```python
from build123d import *

# Parameters (mm, degrees)
MODEL_R             = 5
BOSS_EXTRUDE1_DEPTH = 500


with BuildPart() as part:
    # Model → Boss-Extrude1 (new body)
    with BuildSketch(Plane.XY):
        with BuildLine():
            Line((7.8, 0), (7.8, -4.021825407))
            ThreePointArc((7.8, -4.021825407), (8.10448187, -5.552559136), (8.971572875, -6.850252532))
            Line((8.971572875, -6.850252532), (13.121320343, -11))
            Line((13.121320343, -11), (15.8, -11))
            ThreePointArc((15.8, -11), (16.224264069, -10.824264069), (16.4, -10.4))
            Line((16.4, -10.4), (16.4, -6.8))
            ThreePointArc((16.4, -6.8), (16.575735931, -6.375735931), (17, -6.2))
            Line((17, -6.2), (18.4, -6.2))
            ThreePointArc((18.4, -6.2), (18.824264069, -6.375735931), (19, -6.8))
            Line((19, -6.8), (19, -7.2))
            Line((19, -7.2), (19.4, -7.2))
            ThreePointArc((19.4, -7.2), (19.824264068, -7.375735931), (20, -7.8))
            Line((20, -7.8), (20, -17))
            ThreePointArc((20, -17), (19.121320343, -19.121320343), (17, -20))
            Line((17, -20), (7.8, -20))
            ThreePointArc((7.8, -20), (7.375735931, -19.824264069), (7.2, -19.4))
            ThreePointArc((7.2, -19.4), (7.082842712, -19.117157287), (6.8, -19))
            ThreePointArc((6.8, -19), (6.375735931, -18.824264069), (6.2, -18.4))
            Line((6.2, -18.4), (6.2, -16.999999999))
            ThreePointArc((6.2, -16.999999999), (6.375735931, -16.575735931), (6.8, -16.4))
            Line((6.8, -16.4), (10.4, -16.4))
            ThreePointArc((10.4, -16.4), (10.824264069, -16.224264069), (11, -15.8))
            Line((11, -15.8), (11, -13.369848481))
            ThreePointArc((11, -13.369848481), (10.954327719, -13.140238421), (10.824264069, -12.945584412))
            Line((10.824264069, -12.945584412), (6.850252532, -8.971572875))
            ThreePointArc((6.850252532, -8.971572875), (5.552559136, -8.10448187), (4.021825407, -7.8))
            Line((4.021825407, -7.8), (0, -7.8))
            Line((0, -7.8), (-4.021825407, -7.8))
            ThreePointArc((-4.021825407, -7.8), (-5.552559136, -8.10448187), (-6.850252532, -8.971572875))
            Line((-6.850252532, -8.971572875), (-10.824264069, -12.945584412))
            ThreePointArc((-10.824264069, -12.945584412), (-10.954327719, -13.140238421), (-11, -13.369848481))
            Line((-11, -13.369848481), (-11, -15.8))
            ThreePointArc((-11, -15.8), (-10.824264069, -16.224264069), (-10.4, -16.4))
            Line((-10.4, -16.4), (-6.8, -16.4))
            ThreePointArc((-6.8, -16.4), (-6.375735931, -16.575735931), (-6.2, -16.999999999))
            Line((-6.2, -16.999999999), (-6.2, -18.4))
            ThreePointArc((-6.2, -18.4), (-6.375735931, -18.824264069), (-6.8, -19))
            ThreePointArc((-6.8, -19), (-7.082842712, -19.117157287), (-7.2, -19.4))
            ThreePointArc((-7.2, -19.4), (-7.375735931, -19.824264069), (-7.8, -20))
            Line((-7.8, -20), (-17, -20))
            ThreePointArc((-17, -20), (-19.121320343, -19.121320343), (-20, -17))
            Line((-20, -17), (-20, -7.8))
            ThreePointArc((-20, -7.8), (-19.824264069, -7.375735931), (-19.4, -7.2))
            Line((-19.4, -7.2), (-19, -7.2))
            Line((-19, -7.2), (-19, -6.8))
            ThreePointArc((-19, -6.8), (-18.824264069, -6.375735931), (-18.4, -6.2))
            Line((-18.4, -6.2), (-17, -6.2))
            ThreePointArc((-17, -6.2), (-16.575735931, -6.375735931), (-16.4, -6.8))
            Line((-16.4, -6.8), (-16.4, -10.4))
            ThreePointArc((-16.4, -10.4), (-16.224264069, -10.824264069), (-15.8, -11))
            Line((-15.8, -11), (-13.369848481, -11))
            ThreePointArc((-13.369848481, -11), (-13.140238421, -10.954327719), (-12.945584412, -10.824264069))
            Line((-12.945584412, -10.824264069), (-8.971572875, -6.850252532))
            ThreePointArc((-8.971572875, -6.850252532), (-8.10448187, -5.552559136), (-7.8, -4.021825407))
            Line((-7.8, -4.021825407), (-7.8, 0))
            Line((-7.8, 0), (-7.8, 4.021825407))
            ThreePointArc((-7.8, 4.021825407), (-8.10448187, 5.552559136), (-8.971572875, 6.850252532))
            Line((-8.971572875, 6.850252532), (-12.945584412, 10.824264069))
            ThreePointArc((-12.945584412, 10.824264069), (-13.140238421, 10.954327719), (-13.369848481, 11))
            Line((-13.369848481, 11), (-15.8, 11))
            ThreePointArc((-15.8, 11), (-16.224264069, 10.824264069), (-16.4, 10.4))
            Line((-16.4, 10.4), (-16.4, 6.8))
            ThreePointArc((-16.4, 6.8), (-16.575735931, 6.375735931), (-17, 6.2))
            Line((-17, 6.2), (-18.4, 6.2))
            ThreePointArc((-18.4, 6.2), (-18.824264069, 6.375735931), (-19, 6.8))
            Line((-19, 6.8), (-19, 7.2))
            Line((-19, 7.2), (-19.4, 7.2))
            ThreePointArc((-19.4, 7.2), (-19.824264069, 7.375735931), (-20, 7.8))
            Line((-20, 7.8), (-20, 17))
            ThreePointArc((-20, 17), (-19.121320343, 19.121320343), (-17, 20))
            Line((-17, 20), (-7.8, 20))
            ThreePointArc((-7.8, 20), (-7.375735931, 19.824264068), (-7.2, 19.4))
            Line((-7.2, 19.4), (-7.2, 19))
            Line((-7.2, 19), (-6.8, 19))
            ThreePointArc((-6.8, 19), (-6.375735931, 18.824264069), (-6.2, 18.4))
            Line((-6.2, 18.4), (-6.2, 16.999999999))
            ThreePointArc((-6.2, 16.999999999), (-6.375735931, 16.575735931), (-6.8, 16.4))
            Line((-6.8, 16.4), (-10.4, 16.4))
            ThreePointArc((-10.4, 16.4), (-10.824264069, 16.224264069), (-11, 15.8))
            Line((-11, 15.8), (-11, 13.369848481))
            ThreePointArc((-11, 13.369848481), (-10.954327719, 13.140238421), (-10.824264069, 12.945584412))
            Line((-10.824264069, 12.945584412), (-6.850252532, 8.971572875))
            ThreePointArc((-6.850252532, 8.971572875), (-5.552559136, 8.10448187), (-4.021825407, 7.8))
            Line((-4.021825407, 7.8), (0, 7.8))
            Line((0, 7.8), (4.021825407, 7.8))
            ThreePointArc((4.021825407, 7.8), (5.552559136, 8.10448187), (6.850252532, 8.971572875))
            Line((6.850252532, 8.971572875), (10.824264069, 12.945584412))
            ThreePointArc((10.824264069, 12.945584412), (10.954327719, 13.140238421), (11, 13.369848481))
            Line((11, 13.369848481), (11, 15.8))
            ThreePointArc((11, 15.8), (10.824264069, 16.224264069), (10.4, 16.4))
            Line((10.4, 16.4), (6.8, 16.4))
            ThreePointArc((6.8, 16.4), (6.375735931, 16.575735931), (6.2, 16.999999999))
            Line((6.2, 16.999999999), (6.2, 18.4))
            ThreePointArc((6.2, 18.4), (6.375735931, 18.824264069), (6.8, 19))
            Line((6.8, 19), (7.2, 19))
            Line((7.2, 19), (7.2, 19.4))
            ThreePointArc((7.2, 19.4), (7.375735931, 19.824264068), (7.8, 20))
            Line((7.8, 20), (17, 20))
            ThreePointArc((17, 20), (19.121320343, 19.121320343), (20, 17))
            Line((20, 17), (20, 7.8))
            ThreePointArc((20, 7.8), (19.824264068, 7.375735931), (19.4, 7.2))
            Line((19.4, 7.2), (19, 7.2))
            Line((19, 7.2), (19, 6.8))
            ThreePointArc((19, 6.8), (18.824264069, 6.375735931), (18.4, 6.2))
            Line((18.4, 6.2), (17, 6.2))
            ThreePointArc((17, 6.2), (16.575735931, 6.375735931), (16.4, 6.8))
            Line((16.4, 6.8), (16.4, 10.4))
            ThreePointArc((16.4, 10.4), (16.224264069, 10.824264069), (15.8, 11))
            Line((15.8, 11), (13.369848481, 11))
            ThreePointArc((13.369848481, 11), (13.140238421, 10.954327719), (12.945584412, 10.824264069))
            Line((12.945584412, 10.824264069), (8.971572875, 6.850252532))
            ThreePointArc((8.971572875, 6.850252532), (8.10448187, 5.552559136), (7.8, 4.021825407))
            Line((7.8, 4.021825407), (7.8, 0))
        make_face()
        Circle(MODEL_R, mode=Mode.SUBTRACT)
    extrude(amount=BOSS_EXTRUDE1_DEPTH)


solid = part.part
```
Input: part model. Units: mm. Frame: model coordinates. A direction names the side the tool comes from. Round coordinates to 2 decimals unless told otherwise and drop trailing zeros. Write each question's results on one line, items separated by ' | '.
Q1. Pin query (flat end, axial travel): P1, Ø0.7, axis at y = 17.5, z = 296.5, coming from the +X side; P2, Ø1.5, axis at x = 2, y = 3.5, coming from the -Z side; P3, Ø1, axis at y = -3.5, z = 246, coming from the +X side. Return the tip coordinate at first contact, or that it passes through.
Results:
P1: stops at x = 20 | P2: passes through | P3: stops at x = 7.8
Q2. Line query: line 1 along X through (y, z) = (14.5, 415.5); line 2 along Y through (x, z) = (0, 236); line 3 along X through (y, z) = (-3, 308). Output: solid intervals per line, ascending.
Results:
line 1: x = -20 to -11, 11 to 20 | line 2: y = -7.8 to -5, 5 to 7.8 | line 3: x = -7.8 to -4, 4 to 7.8
Q3. Access query for faces 1 (the face through (-7.8, 0, 246)), 2 (the face through (-12, 20, 246)), 3 (the face through (0, -7.8, 246)). Directions: +Z, -Z, +X, -X, +Y, -Y. A direction counts if a zero-diameter tool reaches every point of the face in a straight line with its end or side. Return the directions, or none.
Results:
face 1: +Z, -Z, -X | face 2: +Z, -Z, +X, -X, +Y | face 3: +Z, -Z, -Y
Q4. Draft query along Y for faces 4 (the face through (20, -12, 246)), 5 (the face through (7.8, 0, 246)), 6 (the face through (0, 7.8, 246)). Return one class per face: released by +Y, released by -Y, zero draft, split by the parting line, or undercut.
Results:
face 4: zero draft | face 5: undercut | face 6: released by +Y
